Here's the drawing with two shaded views (mm, measured from the low corner). I have some questions. Round coordinates to 2 decimals unless told otherwise and drop trailing zeros. Write each loop counter-clockwise with the first axis right and the second up, starting at its lowest first coordinate (ties: lowest second). Pieces come first, ordered by that corner, then holes. Notation, with made-up numbers: M -25.75,25.25 L 19.25,25.25 A6 cw 19.25,36.25 Z; hole C -9.75,-7 d8. An arc over 180 degrees is marked long. Answer as a JSON object with one key per item and string values. Group by question number.
1) Suppose I cut it at C-C, the plane x = 53. Write out the boundary of the cut face in (y, z), and give its area (3 significant figures).
2) Please list where these lines run through material, in increasing order: L1, parallel to Y at x = 53, z = 2.95; L2, parallel to X at y = 18, z = 3.8; L3, parallel to Y at x = 52.5, z = 3.7. Write a range as [from, to].
3) Suppose I cut it at D-D, the plane x = 89. Write out the boundary of the cut face in (y, z), and give its area (3 significant figures).
4) I'm going to push flat-ended pins straight in: pin 1 Ø2 at (y, z) = (6, 1.5) entering from +X; pin 2 Ø1.5 at (y, z) = (20, 3.5) entering from +X. Where does each tip first touch, or does it pass through?
5) Suppose I cut it at B-B, the plane z = 1.8. Write out the boundary of the cut face in (x, y), and give its area (3 significant figures).
6) Suppose I cut it at A-A, the plane y = 5. Write out the boundary of the cut face in (x, z).
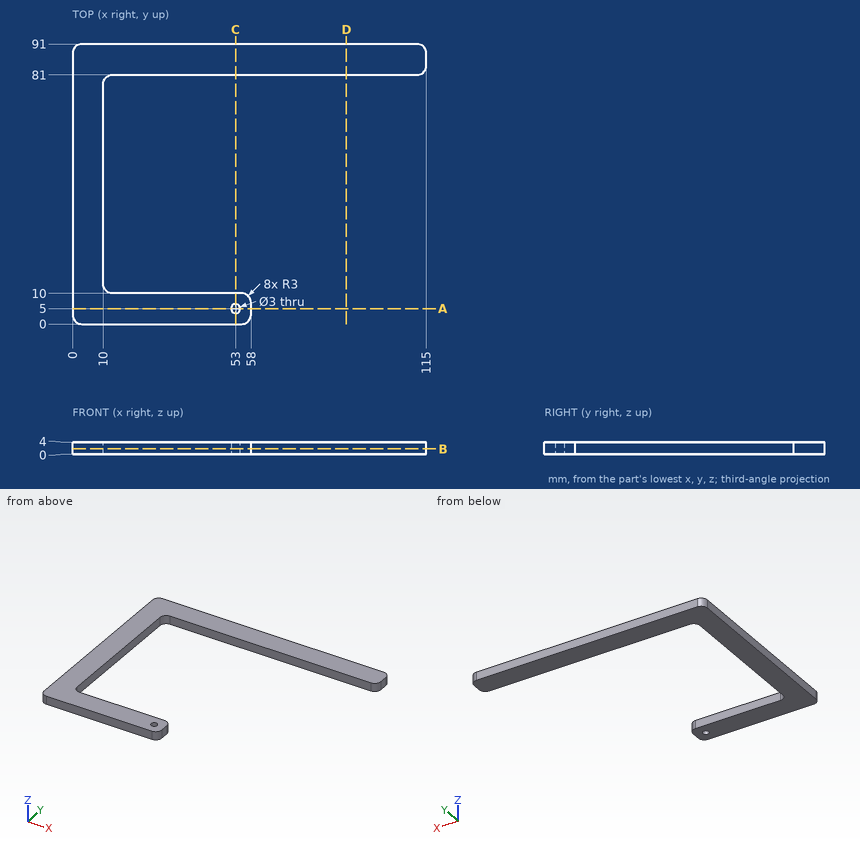
Results:
{
 "1": {"outline": "M 0,0 L 3.5,0 L 3.5,4 L 0,4 Z; M 6.5,0 L 10,0 L 10,4 L 6.5,4 Z; M 81,0 L 91,0 L 91,4 L 81,4 Z", "area": "68.0 mm^2"},
 "2": {"L1": "[0, 3.5], [6.5, 10], [81, 91]", "L2": "[0, 10]", "L3": "[0, 3.59], [6.41, 10], [81, 91]"},
 "3": {"outline": "M 81,0 L 91,0 L 91,4 L 81,4 Z", "area": "40.0 mm^2"},
 "4": {"pin 1": "x = 58", "pin 2": "x = 10"},
 "5": {"outline": "M 0,3 A3 ccw 3,0 L 55,0 A3 ccw 58,3 L 58,7 A3 ccw 55,10 L 13,10 A3 cw 10,13 L 10,78 A3 cw 13,81 L 112,81 A3 ccw 115,84 L 115,88 A3 ccw 112,91 L 3,91 A3 ccw 0,88 Z; hole C 53,5 d3", "area": "2,430 mm^2"},
 "6": {"outline": "M 0,0 L 51.5,0 L 51.5,4 L 0,4 Z; M 54.5,0 L 58,0 L 58,4 L 54.5,4 Z"}
}
